Build history of the part. All positions in model axes, mm. Face numbers are marked on the shaded views. Give positions to 0.01 mm unless a question says otherwise; leave off trailing zeros. Write each loop counter-clockwise with the first axis right and the second up, starting at its lowest first coordinate (ties: lowest second). Pieces come first, ordered by that corner, then holes. Notation, with made-up numbers: M 26,-2.75 L 71,-2.75 A22 ccw 71,32.25 Z; hole C -40,3 d8. An arc over 180 degrees is marked long. Return JSON: item names as keys, results as strings. Group by question number.
Q1. Pull direction X, two halves, no side cores. Call the marked faces 1 and 2: +X half, -X half, draft (parallel to the pull), parting line (faces both ways), or undercut.
Q2. Band-saw the part on C-C, the plane y = 33. Give the cut face in (x, z).
Q3. Flat gauge pins, fed straight in: pin 1 Ø1 at (y, z) = (1, -122.5) entering from -X; pin 2 Ø3 at (x, z) = (-1.5, -103) entering from +Y; pin 3 Ø8 at (x, y) = (-2, 15) entering from +Z. Where does each tip first touch, or does it go through?
Q4. Band-saw the part on B-B, the plane z = -152. Give the cut face in (x, y).
Q5. Band-saw the part on A-A, the plane x = 26. Give the cut face in (y, z), then the cut area to 3 significant figures.
Q6. Wall check: probe 1 along Y at (x, z) = (19, -0.65); probe 2 along Z at (x, y) = (0, 1.55); probe 3 along Y at (x, z) = (0, -167.95). Give the ranges that are in metal, low to high.
Q7. Band-saw the part on D-D, the plane y = 6. Give the cut face in (x, z), then the cut area to 3 significant figures.
from build123d import *

# Parameters (mm, degrees)
EXTRUDE_1_DEPTH     = 50
SKETCH_2_R          = 2.5
CUT_EXTRUDE_1_DEPTH = 58.723478759
SKETCH_3_W          = 4
SKETCH_3_H          = 154
EXTRUDE_2_DEPTH     = 2
SKETCH_4_R          = 5
EXTRUDE_3_DEPTH     = 4
SKETCH_9_R          = 5
EXTRUDE_7_DEPTH     = 4
EXTRUDE_7_2_DEPTH   = 4
EXTRUDE_8_DEPTH     = 2
SKETCH_5_R          = 2.5
CUT_EXTRUDE_3_DEPTH = 182.815875825
SKETCH_11_W         = 4
SKETCH_11_H         = 2
EXTRUDE_9_DEPTH     = 10
SKETCH_12_R         = 5
EXTRUDE_10_DEPTH    = 4
CUT_EXTRUDE_4_REACH = 185.665
SKETCH_13_R         = 2
RIB_2_REACH         = 185.665
SKETCH_15_WALL_W    = 378.061306134
SKETCH_15_WALL_H    = 2
RIB_7_REACH         = 185.665
SKETCH_16_WALL_W    = 379.053421602
SKETCH_16_WALL_H    = 2


with BuildPart() as part:
    # Sketch 1 → Extrude 1 (new body)
    with BuildSketch(Plane(origin=(0, 0, 0), x_dir=(1, 0, 0), z_dir=(0, 1, 0))):
        with BuildLine():
            Line((-14, 0), (-24, 0))
            Line((-24, 0), (-24, 2))
            Line((-24, 2), (-15.874507866, 2))
            ThreePointArc((-15.874507866, 2), (0, 16), (15.874507866, 2))
            Line((15.874507866, 2), (24, 2))
            Line((24, 2), (24, 0))
            Line((24, 0), (14, 0))
            ThreePointArc((14, 0), (0, 14), (-14, 0))
        make_face()
    extrude(amount=EXTRUDE_1_DEPTH)

    # Sketch 2 → Cut-Extrude 1 (cut, through all)
    with BuildSketch(Plane.XY):
        with Locations((-19, 45)):
            Circle(SKETCH_2_R)
        with Locations((-19, 20)):
            Circle(SKETCH_2_R)
    cut_extrude_1 = extrude(amount=-CUT_EXTRUDE_1_DEPTH, mode=Mode.SUBTRACT)

    # Mirror 1: Cut-Extrude 1 across plane
    add(cut_extrude_1.mirror(Plane(origin=(0, 0, 0), x_dir=(0, 0, 1), z_dir=(1, 0, 0))), mode=Mode.SUBTRACT)

    # Sketch 3 → Extrude 2 (add)
    with BuildSketch(Plane(origin=(0, 0, 0), x_dir=(1, 0, 0), z_dir=(0, 1, 0))):
        with Locations((0, 91)):
            Rectangle(SKETCH_3_W, SKETCH_3_H)
    extrude(amount=EXTRUDE_2_DEPTH)

    # Sketch 4 → Extrude 3 (add)
    with BuildSketch(Plane(origin=(0, 0, 0), x_dir=(1, 0, 0), z_dir=(0, 1, 0))):
        with Locations(Location((0, 52, 0), (0, 0, 113.578178478))):
            Circle(SKETCH_4_R)
        with Locations(Location((0, 102, 0), (0, 0, 66.421821522))):
            Circle(SKETCH_4_R)
        with Locations(Location((0, 152, 0), (0, 0, 66.421821522))):
            Circle(SKETCH_4_R)
    extrude(amount=EXTRUDE_3_DEPTH)



with BuildPart() as body_2:
    # Sketch 9 → Extrude 7 (new body)
    with BuildSketch(Plane(origin=(0, 0, 0), x_dir=(1, 0, 0), z_dir=(0, 1, 0))):
        with Locations(Location((-43.301270189, 77, 0), (0, 0, 270))):
            Circle(SKETCH_9_R)
    extrude(amount=EXTRUDE_7_DEPTH)


with BuildPart() as body_3:
    # Sketch 9 → Extrude 7 2 (new body)
    with BuildSketch(Plane(origin=(0, 0, 0), x_dir=(1, 0, 0), z_dir=(0, 1, 0))):
        with Locations(Location((43.301270189, 77, 0), (0, 0, 90))):
            Circle(SKETCH_9_R)
    extrude(amount=EXTRUDE_7_2_DEPTH)


with BuildPart() as part_1:
    add(part.part)

    add(body_2.part)  # Extrude 8 merges body 2

    add(body_3.part)  # Extrude 8 merges body 3
    # Sketch 10 → Extrude 8 (add)
    with BuildSketch(Plane(origin=(0, 0, 0), x_dir=(1, 0, 0), z_dir=(0, 1, 0))):
        Polygon((0, 104.309401077), (-47.301270189, 77), (0, 49.690598923), (47.301270189, 77), align=None)
        Polygon((0, 99.690598923), (-39.301270189, 77), (0, 54.309401077), (39.301270189, 77), align=None, mode=Mode.SUBTRACT)
    extrude(amount=EXTRUDE_8_DEPTH)

    # Sketch 5 → Cut-Extrude 3 (cut, through all)
    with BuildSketch(Plane(origin=(0, 0, 0), x_dir=(1, 0, 0), z_dir=(0, 1, 0))):
        with Locations(Location((0, 102, 0), (0, 0, 270))):
            Circle(SKETCH_5_R)
        with Locations(Location((0, 52, 0), (0, 0, 270))):
            Circle(SKETCH_5_R)
        with Locations(Location((0, 152, 0), (0, 0, 270))):
            Circle(SKETCH_5_R)
        with Locations(Location((-43.301270189, 77, 0), (0, 0, 270))):
            Circle(SKETCH_5_R)
        with Locations(Location((43.301270189, 77, 0), (0, 0, 90))):
            Circle(SKETCH_5_R)
    extrude(amount=CUT_EXTRUDE_3_DEPTH, mode=Mode.SUBTRACT)

    # Sketch 11 → Extrude 9 (add)
    with BuildSketch(Plane(origin=(0, 0, 0), x_dir=(1, 0, 0), z_dir=(0, 1, 0))):
        with Locations((0, 169)):
            Rectangle(SKETCH_11_W, SKETCH_11_H)
    extrude(amount=EXTRUDE_9_DEPTH)

    # Sketch 12 → Extrude 10 (add)
    with BuildSketch(Plane(origin=(0, 0, -170), x_dir=(-1, 0, 0), z_dir=(0, 0, -1))):
        with Locations((0, 14)):
            Circle(SKETCH_12_R)
    extrude(amount=-EXTRUDE_10_DEPTH)

    # Sketch 13 → Cut-Extrude 4 (cut, up to next)
    with BuildSketch(Plane(origin=(0, 0, -170), x_dir=(-1, 0, 0), z_dir=(0, 0, -1)), mode=Mode.PRIVATE) as cut_extrude_4_sk1:
        with Locations((0, 14)):
            Circle(SKETCH_13_R)
    cut_extrude_4_tool1 = extrude(cut_extrude_4_sk1.sketch, amount=-CUT_EXTRUDE_4_REACH, mode=Mode.PRIVATE) & part_1.part
    add(cut_extrude_4_tool1.solids().sort_by_distance((0, 14, -170))[0], mode=Mode.SUBTRACT)

    # Sketch 15 wall → Rib 2 (add, up to next)
    with BuildSketch(Plane(origin=(0, 5.650617497, -163.373503951), x_dir=(0, -0.707106781187, 0.707106781187), z_dir=(0, -0.707106781187, -0.707106781187)), mode=Mode.PRIVATE) as rib_2_sk1:
        Rectangle(SKETCH_15_WALL_W, SKETCH_15_WALL_H)
    rib_2_tool1 = extrude(rib_2_sk1.sketch, amount=RIB_2_REACH, mode=Mode.PRIVATE) - part_1.part
    add(rib_2_tool1.solids().sort_by_distance((0, 5.650617497, -163.373503951))[0])

    # Sketch 16 wall → Rib 7 (add, up to next)
    with BuildSketch(Plane(origin=(0, 6.071182812, -19.696276491), x_dir=(0, -0.707106781187, -0.707106781187), z_dir=(0, 0.707106781187, -0.707106781187)), mode=Mode.PRIVATE) as rib_7_sk1:
        Rectangle(SKETCH_16_WALL_W, SKETCH_16_WALL_H)
    rib_7_tool1 = extrude(rib_7_sk1.sketch, amount=-RIB_7_REACH, mode=Mode.PRIVATE) - part_1.part
    add(rib_7_tool1.solids().sort_by_distance((0, 6.071182812, -19.696276491))[0])


solid = part_1.part
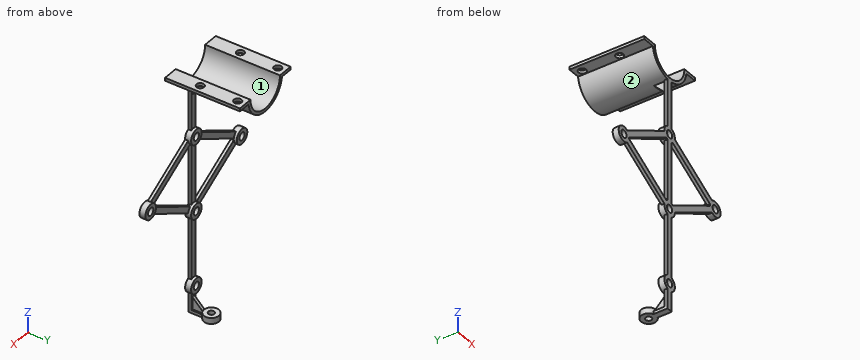
From the geometry:
{
 "1": {"face 1": "undercut", "face 2": "parting line"},
 "2": {"outline": "M -24,-2 L -15.87,-2 A16 ccw 15.87,-2 L 24,-2 L 24,0 L 14,0 A14 cw -14,0 L -24,0 Z"},
 "3": {"pin 1": "stops at x = -2", "pin 2": "stops at y = 4", "pin 3": "stops at z = -12.65"},
 "4": {"outline": "M -5,0 L -2.5,0 L -2.5,4 L -5,4 Z; M 2.5,0 L 5,0 L 5,4 L 2.5,4 Z"},
 "5": {"outline": "M 0,-89.3 L 2,-89.3 L 2,-84.68 L 0,-84.68 Z; M 0,-69.32 L 2,-69.32 L 2,-64.7 L 0,-64.7 Z", "area": "18.5 mm^2"},
 "6": {"probe 1": "y = 0 to 17.5, 22.5 to 42.5, 47.5 to 50", "probe 2": "z = -170 to -154.5, -149.5 to -104.5, -99.5 to -54.5, -49.5 to -14", "probe 3": "y = 0 to 12, 16 to 19"},
 "7": {"outline": "M -24,-2 L -15.87,-2 A16 ccw -1,-15.97 L -1,-19.77 L 1,-19.77 L 1,-15.97 A16 ccw 15.87,-2 L 24,-2 L 24,0 L 14,0 A14 cw -14,0 L -24,0 Z; M -2,-170 L 2,-170 L 2,-168 L 1,-168 L 1,-163.72 L -1,-163.72 L -1,-168 L -2,-168 Z", "area": "151 mm^2"}
}
